Check sheet for the modelled part. Datum: model origin and axes. Units: mm. Face numbers are marked on the shaded views. A direction names the side the tool comes from. Round coordinates to 2 decimals unless told otherwise and drop trailing zeros. Loops run counter-clockwise (first coordinate to the right, second up) from the corner with the lowest first, then second, coordinate; pieces in that order, holes last. Notation, with made-up numbers: (12, -3) - (60, -3) arc R20 cw to (60, 26) - close; hole circle Ø8 at (81.25, 44). An arc over 180 degrees is marked (long way). Put each result on its own line as item: value. Start each with the question number.
Item 1: Section check D-D, the plane y = 7.5. Record the cut outline in (x, z), and give its area (3 significant figures).
Item 2: Section check A-A, the plane x = -1. Record the cut outline in (y, z), and give its area (3 significant figures).
Item 3: Section check C-C, the plane z = 5.5. Record the cut outline in (x, y), and give its area (3 significant figures).
Item 4: Draft check along Y on the marked faces 5, 6 and 7. Enter one of: pulls with the +Y half, pulls with the -Y half, needs draft (parallel to the pull), parting line crosses it, or undercut.
Item 5: Gauge pin test, flat ends, axial feed: pin 1 Ø2 at (y, z) = (5, 4.5) entering from +X; pin 2 Ø5 at (y, z) = (23, -4.5) entering from -X; pin 3 Ø2 at (y, z) = (29.5, -3.5) entering from -X. Record the tip position at first contact, or that the pin passes through.
Item 6: Section check B-B, the plane y = 20.5. Record the cut outline in (x, z), and give its area (3 significant figures).
Item 7: Tool access check on the marked faces 1, 2, 3 and 4. Record the directions out of +Z, -Z, +X, -X, +Y, -Y that give a thin tool (end or side, any length) a straight path to the whole face; none if there is none.
Item 8: Material ranges on line 1 along Y through (x, z) = (6.55, 0); line 2 along X through (y, z) = (13.25, 0); line 3 along Y through (x, z) = (2.75, -5), recorded low to high.
from build123d import *

# Parameters (mm, degrees)
SKETCH1_R           = 8
BOSS_EXTRUDE1_DEPTH = 5
SKETCH2_R           = 6.1
BOSS_EXTRUDE2_DEPTH = 9
SKETCH3_R           = 6.1
BOSS_EXTRUDE3_DEPTH = 17
SKETCH4_R           = 6.1
BOSS_EXTRUDE4_DEPTH = 9
CUT_EXTRUDE1_START  = -4
CUT_EXTRUDE1_DEPTH  = 4
CUT_EXTRUDE2_DEPTH  = 4
SKETCH7_R           = 6.1
BOSS_EXTRUDE5_DEPTH = 11
CUT_EXTRUDE3_DEPTH  = 8
SKETCH9_R           = 3.15
CUT_EXTRUDE4_DEPTH  = 25
SKETCH10_R          = 1.5
CUT_EXTRUDE5_DEPTH  = 53.239831546
SKETCH11_R          = 1.5
CUT_EXTRUDE6_DEPTH  = 6


with BuildPart() as part:
    # Sketch1 → Boss-Extrude1 (new body)
    with BuildSketch(Plane(origin=(0, 0, 0), x_dir=(1, 0, 0), z_dir=(0, 1, 0))):
        with Locations(Location((0, 0, 0), (0, 0, 270))):
            Circle(SKETCH1_R)
    extrude(amount=BOSS_EXTRUDE1_DEPTH)

    # Sketch2 → Boss-Extrude2 (add)
    with BuildSketch(Plane(origin=(0, 5, 0), x_dir=(1, 0, 0), z_dir=(0, 1, 0))):
        with Locations(Location((1, 0, 0), (0, 0, 270))):
            Circle(SKETCH2_R)
    extrude(amount=BOSS_EXTRUDE2_DEPTH)

    # Sketch3 → Boss-Extrude3 (add)
    with BuildSketch(Plane(origin=(0, 14, 0), x_dir=(1, 0, 0), z_dir=(0, 1, 0))):
        with Locations(Location((-1, 0, 0), (0, 0, 80.564661277))):
            Circle(SKETCH3_R)
    extrude(amount=BOSS_EXTRUDE3_DEPTH)

    # Sketch4 → Boss-Extrude4 (add)
    with BuildSketch(Plane(origin=(0, 31, 0), x_dir=(1, 0, 0), z_dir=(0, 1, 0))):
        with Locations(Location((1, 0, 0), (0, 0, 99.435338723))):
            Circle(SKETCH4_R)
    extrude(amount=BOSS_EXTRUDE4_DEPTH)

    # Sketch5 → Cut-Extrude1 (cut)
    with BuildSketch(Plane(origin=(0, 31, 0), x_dir=(1, 0, 0), z_dir=(0, 1, 0)).offset(CUT_EXTRUDE1_START)):
        with BuildLine():
            ThreePointArc((0, 6.017474553), (-5.1, 0), (0, -6.017474553))
            ThreePointArc((0, -6.017474553), (-7.1, 0), (0, 6.017474553))
        make_face()
    extrude(amount=CUT_EXTRUDE1_DEPTH, mode=Mode.SUBTRACT)

    # Sketch6 → Cut-Extrude2 (cut)
    with BuildSketch(Plane.XZ.offset(-14)):
        with BuildLine():
            ThreePointArc((0, 6.017474553), (-7.1, 0), (0, -6.017474553))
            ThreePointArc((0, -6.017474553), (-5.1, 0), (0, 6.017474553))
        make_face()
    extrude(amount=-CUT_EXTRUDE2_DEPTH, mode=Mode.SUBTRACT)

    # Sketch7 → Boss-Extrude5 (add)
    with BuildSketch(Plane(origin=(0, 40, 0), x_dir=(1, 0, 0), z_dir=(0, 1, 0))):
        with Locations(Location((0, 0, 0), (0, 0, 85.298349803))):
            Circle(SKETCH7_R)
    extrude(amount=BOSS_EXTRUDE5_DEPTH)

    # Sketch8 → Cut-Extrude3 (cut)
    with BuildSketch(Plane.XZ.offset(-40)):
        with BuildLine():
            ThreePointArc((0.5, 6.079473661), (-6.1, 0), (0.5, -6.079473661))
            ThreePointArc((0.5, -6.079473661), (-5.1, 0), (0.5, 6.079473661))
        make_face()
    extrude(amount=-CUT_EXTRUDE3_DEPTH, mode=Mode.SUBTRACT)

    # Sketch9 → Cut-Extrude4 (cut)
    with BuildSketch(Plane.XZ):
        with Locations(Location((0, 0, 0), (0, 0, 270))):
            Circle(SKETCH9_R)
    extrude(amount=-CUT_EXTRUDE4_DEPTH, mode=Mode.SUBTRACT)

    # Sketch10 → Cut-Extrude5 (cut, through all)
    with BuildSketch(Plane(origin=(0, 0, 0), x_dir=(0, 0, -1), z_dir=(1, 0, 0))):
        with Locations(Location((0, 7.5, 0), (0, 0, 180))):
            Circle(SKETCH10_R)
    extrude(amount=CUT_EXTRUDE5_DEPTH, mode=Mode.SUBTRACT)

    # Sketch11 → Cut-Extrude6 (cut)
    with BuildSketch(Plane(origin=(0, 0, 0), x_dir=(0, 0, -1), z_dir=(1, 0, 0))):
        Polygon((0, 10.733161507), (-2.8, 9.116580754), (-2.8, 5.883419246), (0, 4.266838493), (2.8, 5.883419246), (2.8, 9.116580754), align=None)
        with Locations(Location((0, 7.5, 0), (0, 0, 180))):
            Circle(SKETCH11_R, mode=Mode.SUBTRACT)
    extrude(amount=CUT_EXTRUDE6_DEPTH, mode=Mode.SUBTRACT)


solid = part.part
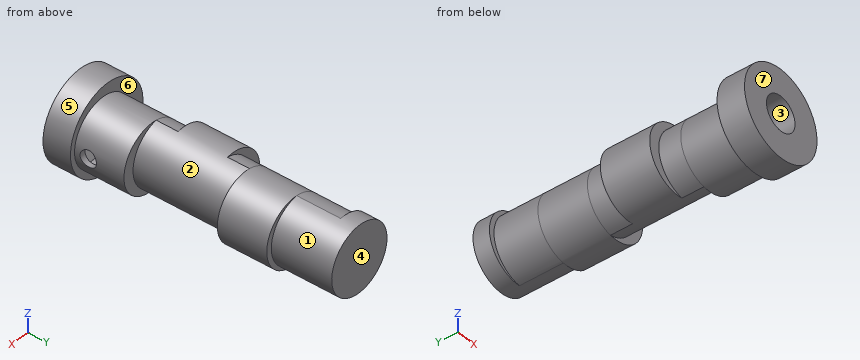
Check result:
1. outline: (1.44, -2.8) arc R3.15 cw (long way) to (1.44, 2.8) - (6, 2.8) - (6, 1.5) - (6.91, 1.5) arc R6.1 ccw (long way) to (6.91, -1.5) - (6, -1.5) - (6, -2.8) - close
1. area: 63.9 mm²
2. outline: (0, -7.94) - (5, -7.94) - (5, -5.76) - (18, -5.76) - (18, -6.1) - (27, -6.1) - (27, -5.76) - (48, -5.76) - (48, -6.02) - (51, -6.02) - (51, 6.02) - (48, 6.02) - (48, 5.76) - (27, 5.76) - (27, 6.1) - (18, 6.1) - (18, 5.76) - (5, 5.76) - (5, 7.94) - (0, 7.94) - (0, 2.99) - (25, 2.99) - (25, -2.99) - (0, -2.99) - close
2. area: 468 mm²
3. outline: (-5.81, 0) - (5.81, 0) - (5.81, 5) - (3.64, 5) - (3.64, 14) - (1.64, 14) - (1.64, 31) - (3.64, 31) - (3.64, 40) - (2.64, 40) - (2.64, 51) - (-2.64, 51) - (-2.64, 48) - (-1.64, 48) - (-1.64, 27) - (-3.64, 27) - (-3.64, 18) - (-1.64, 18) - (-1.64, 5) - (-5.81, 5) - close
3. area: 277 mm²
4. face 5: needs draft
4. face 6: undercut
4. face 7: pulls with the -Y half
5. pin 1: x = 7.19
5. pin 2: x = -6.76
5. pin 3: x = -4.56
6. outline: circle Ø12.2 at (-1, 0); hole circle Ø6.3 at (0, 0)
6. area: 85.7 mm²
7. face 1: +Y
7. face 2: none
7. face 3: -Y
7. face 4: +Z, -Z, +X, -X, +Y
8. line 1: 0 to 6, 9 to 14, 31 to 40
8. line 2: -5.1 to -3.15, 3.15 to 7.1
8. line 3: 0 to 14, 31 to 51
